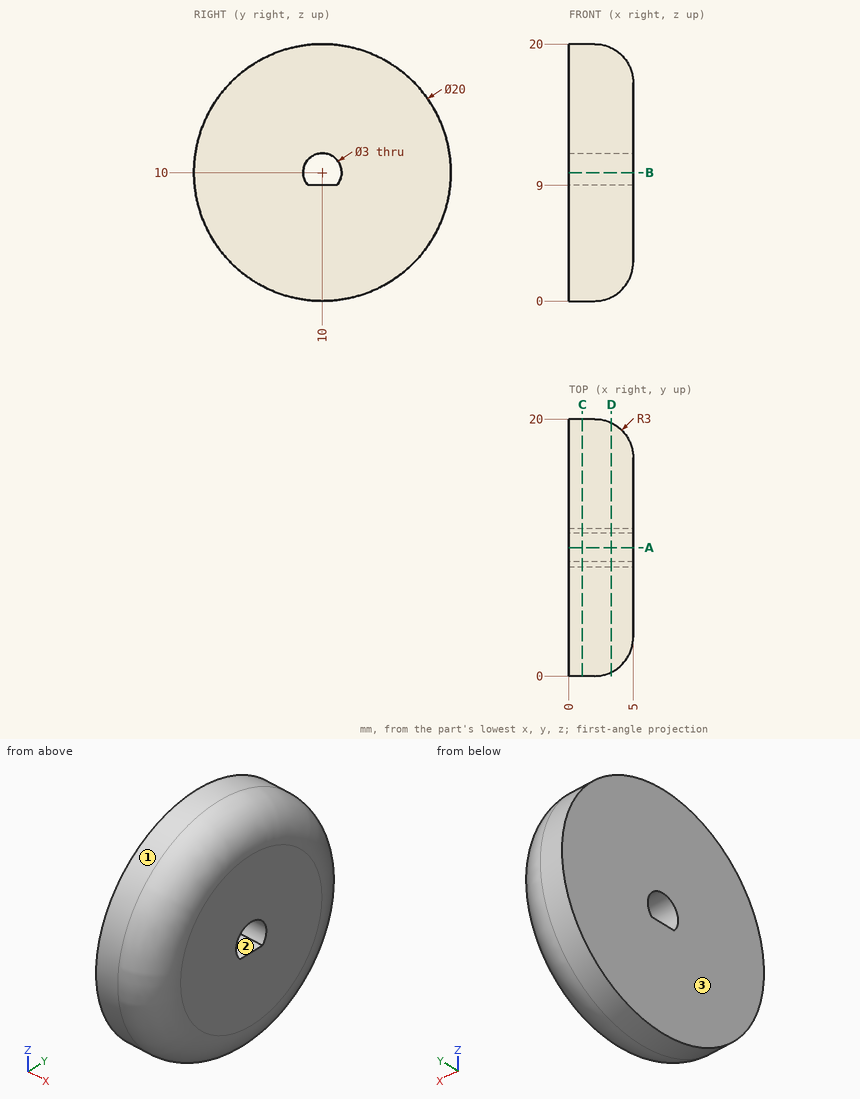
Print and shaded views of the part. All mm, measured from the part's lowest x, y and z. Give positions to 0.01 mm unless a question says otherwise; leave off trailing zeros. Loops run counter-clockwise (first coordinate to the right, second up) from the corner with the lowest first, then second, coordinate; pieces in that order, holes last. Notation, with made-up numbers: (31.5, -11) -> (53.5, -11) arc R37 ccw to (53.5, 25) -> close; hole circle Ø7 at (41, 8). An arc over 180 degrees is marked (long way). One line per question, with ' | ' between items. Start each with the question number.
1) Probe L1, parallel to Z at x = 1.7, y = 10; L2, parallel to Y at x = 1.5, z = 10; L3, parallel to Y at x = 3.8, z = 10. List the from-to ranges inside material, lowest first.
2) Cut at D-D (x = 3.3). Give the cut face in (y, z).
3) Pin check, flat tips, straight feed: pin 1 (3 mm diameter, centred on x = 4, y = 17, fed in from -Z); pin 2 (0.7 mm diameter, centred on x = 3, y = 9.5, fed in from +Z); pin 3 (1.5 mm diameter, centred on x = 3.5, z = 15, fed in from +Y). Stop position of each tip, or through.
4) Cut at A-A (y = 10). Give the cut face in (x, z), plus the area to 3 significant figures.
5) Cut at B-B (z = 10). Give the cut face in (x, y), plus the area to 3 significant figures.
6) Two-plate mould, pull along Y, no slides. Class the marked faces 1, 2 and 3: released by +Y, released by -Y, zero draft, split by the parting line, or undercut.
7) Cut at C-C (x = 1.05). Give the cut face in (y, z).
Return value:
1) L1: 0 to 9, 11.5 to 20 | L2: 0 to 8.5, 11.5 to 20 | L3: 0.6 to 8.5, 11.5 to 19.4
2) outline: circle Ø19.41 at (10, 10); hole (8.88, 9) -> (11.12, 9) arc R1.5 ccw (long way) to start
3) pin 1: z = 2.11 | pin 2: z = 19.92 | pin 3: y = 18.77
4) outline: (0, 0) -> (2, 0) arc R3 ccw to (5, 3) -> (5, 9) -> (0, 9) -> close; (0, 11.5) -> (5, 11.5) -> (5, 17) arc R3 ccw to (2, 20) -> (0, 20) -> close | area: 83.6 mm^2
5) outline: (0, 0) -> (2, 0) arc R3 ccw to (5, 3) -> (5, 8.5) -> (0, 8.5) -> close; (0, 11.5) -> (5, 11.5) -> (5, 17) arc R3 ccw to (2, 20) -> (0, 20) -> close | area: 81.1 mm^2
6) face 1: split by the parting line | face 2: undercut | face 3: zero draft
7) outline: circle Ø20 at (10, 10); hole (8.88, 9) -> (11.12, 9) arc R1.5 ccw (long way) to start
